```python
from build123d import *

# Parameters (mm, degrees)
F1_DEPTH = 12.7
F2_DEPTH = 76.2
F4_DEPTH = 12.7
F3_W     = 19.05
F3_H     = 19.05
F5_DEPTH = 25.4


# Not quite as in the source:
# - a feature names something its author has since deleted; it is built from what else it names


with BuildPart() as f1:
    # F0 (on Top) → F1 (new body)
    with BuildSketch(Plane.XY):
        with BuildLine():
            Line((59.8826112453, 4.7625), (-73.4673887547, 4.7625))
            ThreePointArc((-73.4673887547, 4.7625), (-82.9923886673, -4.7625000437), (-73.4673886673, -14.2875))
            Line((-73.4673886673, -14.2875), (59.9451471992, -14.2875))
            Line((59.9451471992, -14.2875), (59.8826112453, 4.7625))
        make_face()
        Polygon((78.9326112453, 4.7625), (59.8826112453, 4.7625), (59.9451471992, -14.2875), (78.9326113327, -14.2875), align=None)
    extrude(amount=F1_DEPTH)

    # F0 (on Top) → F2 (join)
    with BuildSketch(Plane.XY):
        Polygon((78.9326112453, 4.7625), (59.8826112453, 4.7625), (59.9451471992, -14.2875), (78.9326113327, -14.2875), align=None)
    extrude(amount=F2_DEPTH)

    # F3 (on face) → F4 (join)
    with BuildSketch(Plane.XY.offset(76.2)):
        Polygon((78.9326113327, -14.2875), (59.9451471992, -14.2875), (59.9451471992, -223.8375), (78.9951471992, -223.8375), (78.9951471992, -14.2875), align=None)
    extrude(amount=-F4_DEPTH)

    # F3 (on face) → F5 (join)
    with BuildSketch(Plane.XY.offset(76.2)):
        with Locations((69.4701471992, -233.3625)):
            Rectangle(F3_W, F3_H)
    extrude(amount=-F5_DEPTH)


with BuildPart() as f6_1:
    # F6: copy of F1
    add(f1.part)


solid = f1.part
```
Check sheet for the modelled part. Datum: model origin and axes. Units: mm. A direction names the side the tool comes from. Round coordinates to 2 decimals unless told otherwise and drop trailing zeros. Write each loop counter-clockwise with the first axis right and the second up, starting at its lowest first coordinate (ties: lowest second). Pieces come first, ordered by that corner, then holes. Notation, with made-up numbers: M -35.5,4 L 22.5,4 A25 ccw 22.5,26 Z; hole C 64.5,-34 d2. An arc over 180 degrees is marked long. Write item = value, one per line. Start each with the question number.
1. Section check D-D, the plane x = 20.5. Record the cut outline in (y, z), then the cut area to 3 significant figures.
2. Section check B-B, the plane z = 69. Record the cut outline in (x, y).
3. Section check C-C, the plane y = -143. Record the cut outline in (x, z), then the cut area to 3 significant figures.
4. Scan lines: line 1 (X direction, y = -64, z = 67); line 2 (Z direction, x = 34.5, y = -9.5); line 3 (Z direction, x = 65, y = -22). Record each from-to range of solid material in increasing order. Write a range as [from, to].
5. Gauge pin test, flat ends, axial feed: pin 1 (9.5 mm diameter, centred on y = -8, z = 38.5, fed in from +X); pin 2 (15 mm diameter, centred on x = 66.5, y = -134, fed in from -Z); pin 3 (12.5 mm diameter, centred on y = -134.5, z = 69, fed in from -X). Record the tip position at first contact, or that the pin passes through.
6. Tool access check on faces 1 (the flat face through (69, -118, 63.5)), 2 (the flat face through (-13, -5, 12.7)). Record the directions out of +Z, -Z, +X, -X, +Y, -Y that give a thin tool (end or side, any length) a straight path to the whole face; none if there is none.
7. Section check A-A, the plane z = 54. Record the cut outline in (x, y).
8. Release check for a two-part mould opening along Y. For faces 3 (the flat face through (69, -233, 50.8)), 4 (the cylindrical face through (-82.99, -4.55, 6.26)), 5 (the flat face through (69, -223.838, 57)), 6 (the flat face through (20, 4.762, 12.5)) record: pulls with the +Y half, pulls with the -Y half, needs draft (parallel to the pull), parting line crosses it, or undercut.
Results found:
q1.outline = M -14.29,0 L 4.76,0 L 4.76,12.7 L -14.29,12.7 Z
q1.area = 242 mm^2
q2.outline = M 59.88,4.76 L 59.95,-14.29 L 59.95,-242.89 L 79,-242.89 L 79,-14.29 L 78.93,-14.29 L 78.93,4.76 Z
q3.outline = M 59.95,63.5 L 79,63.5 L 79,76.2 L 59.95,76.2 Z
q3.area = 242 mm^2
q4.line_1 = [59.95, 79]
q4.line_2 = [0, 12.7]
q4.line_3 = [63.5, 76.2]
q5.pin_1 = 78.93
q5.pin_2 = 63.5
q5.pin_3 = 59.95
q6.face_1 = -Z, +X, -X
q6.face_2 = +Z, -X, +Y, -Y
q7.outline = M 59.88,4.76 L 59.95,-14.29 L 78.93,-14.29 L 78.93,4.76 Z; M 59.95,-242.89 L 79,-242.89 L 79,-223.84 L 59.95,-223.84 Z
q8.face_3 = needs draft
q8.face_4 = parting line crosses it
q8.face_5 = undercut
q8.face_6 = pulls with the +Y half
